Work out the finished part from the listing and answer in its coordinate system (mm). Face numbers are marked on the shaded views. A direction names the side the tool comes from. Give positions to 0.01 mm unless a question says otherwise; leave off trailing zeros. Order: outer loops, then holes, each group sorted by start corner. A loop starts at its lowest first (then second) coordinate and runs counter-clockwise, first axis right, second up.
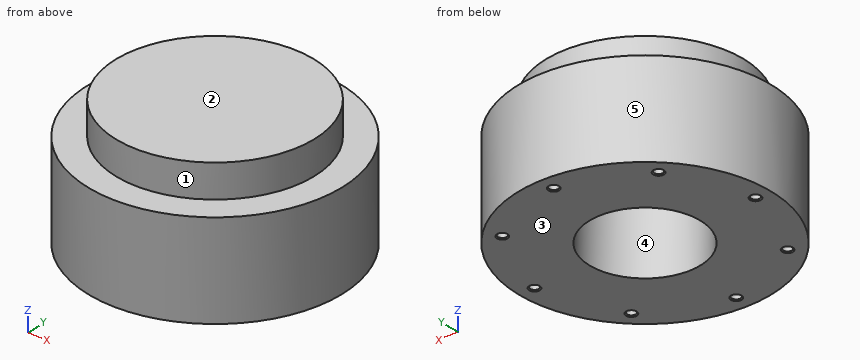
```python
from build123d import *

# Parameters (mm, degrees)
SKETCH1_R                   = 37.5
SKETCH1_R_2                 = 21
BOSS_EXTRUDE1_DEPTH         = 12.5
BOSS_EXTRUDE2_START         = -36
SKETCH1_3_R                 = 48
SKETCH1_3_R_2               = 37.5
SKETCH1_3_R_3               = 21
BOSS_EXTRUDE2_DEPTH         = 36
M4_TAPPED_HOLE1_D           = 3.3
M4_TAPPED_HOLE1_DEPTH       = 8
M4_TAPPED_HOLE1_CSINK_D     = 4.05
M4_TAPPED_HOLE1_CSINK_ANGLE = 90
M4_TAPPED_HOLE1_TIP         = 0.991420021


with BuildPart() as part:
    # Sketch1 → Boss-Extrude1 (new body)
    # profile 1 of 2: a face of its own
    with BuildSketch(Plane.XY):
        Circle(SKETCH1_R)
        Circle(SKETCH1_R_2, mode=Mode.SUBTRACT)
    # profile 2 of 2: a face of its own
    with BuildSketch(Plane.XY):
        Circle(SKETCH1_R_2)
    extrude(amount=BOSS_EXTRUDE1_DEPTH)

    # Sketch1_3 → Boss-Extrude2 (add)
    # profile 1 of 2: a face of its own
    with BuildSketch(Plane.XY.offset(BOSS_EXTRUDE2_START)):
        Circle(SKETCH1_3_R)
        Circle(SKETCH1_3_R_2, mode=Mode.SUBTRACT)
    # profile 2 of 2: a face of its own
    with BuildSketch(Plane.XY.offset(BOSS_EXTRUDE2_START)):
        Circle(SKETCH1_3_R_2)
        Circle(SKETCH1_3_R_3, mode=Mode.SUBTRACT)
    extrude(amount=BOSS_EXTRUDE2_DEPTH)

    # M4 Tapped Hole1
    with Locations(Plane(origin=(0, 0, -36), x_dir=(-1, 0, 0), z_dir=(0, 0, -1))):
        with Locations((0, 42), (29.69848481, 29.69848481), (42, 0), (29.69848481, -29.69848481), (0, -42), (-29.69848481, -29.69848481), (-42, 0), (-29.69848481, 29.69848481)):
            CounterSinkHole(M4_TAPPED_HOLE1_D / 2, M4_TAPPED_HOLE1_CSINK_D / 2, depth=M4_TAPPED_HOLE1_DEPTH, counter_sink_angle=M4_TAPPED_HOLE1_CSINK_ANGLE)
            with Locations((0, 0, -(M4_TAPPED_HOLE1_DEPTH + M4_TAPPED_HOLE1_TIP / 2))):  # 118° drill point
                Cone(0, M4_TAPPED_HOLE1_D / 2, M4_TAPPED_HOLE1_TIP, mode=Mode.SUBTRACT)


solid = part.part
```
1. Given P1, Ø1, axis at x = -27, z = 1, coming from the +Y side; P2, Ø2, axis at x = -29.7, y = -29.7, coming from the +Z side; P3, Ø5, axis at x = -28, z = -21, coming from the -Y side, each flat-ended and moving along its own axis, determine where each tip first touches the part or whether it passes through.
Findings below:
P1: stops at y = 26.53
P2: stops at z = 0
P3: stops at y = -40.67
2. The mould has two halves that part along X. Classify the marked faces 3, 4 and 5: pulls with the +X half, pulls with the -X half, needs draft (parallel to the pull), parting line crosses it, or undercut.
Findings below:
face 3: needs draft
face 4: undercut
face 5: parting line crosses it
3. Straight lines are drawn through the part: probe 1 along Y at (x, z) = (0, -32); probe 2 along X at (y, z) = (0.5, -12.5); probe 3 along Z at (x, y) = (-4.5, -4.5). For each, find the intervals that lie inside material, in ascending order.
Findings below:
probe 1: y = -48 to -43.65, -40.35 to -21, 21 to 40.35, 43.65 to 48
probe 2: x = -48 to -20.99, 20.99 to 48
probe 3: z = 0 to 12.5
4. The part is cut by section B-B (y = 8). Write down the section's boundary in (x, z).
Findings below:
outline: (-47.33, -36) - (-19.42, -36) - (-19.42, 0) - (19.42, 0) - (19.42, -36) - (47.33, -36) - (47.33, 0) - (36.64, 0) - (36.64, 12.5) - (-36.64, 12.5) - (-36.64, 0) - (-47.33, 0) - close
5. The part is cut by section D-D (x = 10). Write down the section's boundary in (y, z).
Findings below:
outline: (-46.95, -36) - (-18.47, -36) - (-18.47, 0) - (18.47, 0) - (18.47, -36) - (46.95, -36) - (46.95, 0) - (36.14, 0) - (36.14, 12.5) - (-36.14, 12.5) - (-36.14, 0) - (-46.95, 0) - close
6. The part is cut by section A-A (z = -32). State how many separate pieces and enclosed holes the cut face has, then the cut area to 3 significant figures.
Findings below:
separate pieces: 1
enclosed holes: 9
area: 5,780 mm2
7. The part is cut by section C-C (z = -25.5). Write down the section's boundary in (x, y), then the cut area to 3 significant figures.
Findings below:
outline: circle Ø96 at (0, 0); hole circle Ø42 at (0, 0)
area: 5,850 mm2
8. Which of the six approach directions +Z, -Z, +X, -X, +Y, -Y give full straight-line access (tool end or side, diameter ignored) to the marked faces 1 and 2?
Findings below:
face 1: +Z
face 2: +Z, +X, -X, +Y, -Y
